Check sheet for the modelled part. Datum: model origin and axes. Units: mm. Round coordinates to 2 decimals unless told otherwise and drop trailing zeros. Answer in a Markdown table with one row per item. Add a question column.
(1) Thickness scan on line 1 along X through (y, z) = (250, -2.9); line 2 along Y through (x, z) = (15, -2.9). Record the ranges inside material, lowest first.
(2) Gauge pin test, flat ends, axial feed: pin 1 (6.5 mm diameter, centred on x = 15, y = 50, fed in from -Z); pin 2 (6.5 mm diameter, centred on x = 15, y = 450, fed in from +Z). Record the tip position at first contact, or that the pin passes through.
(3) Mould release check, pull along Y, two halves, no side actions. Record for faces 1 (the flat face through (217, 254, -3)), 2 (the conical face through (15.63, 47.18, -2.71)): +Y half, -Y half, draft (parallel to the pull), parting line (faces both ways), or undercut.
from build123d import *

# Parameters (mm, degrees)
F0_W           = 440
F0_H           = 500
F1_DEPTH       = 3
F2_D           = 5.5
F2_CSINK_D     = 11.2
F2_CSINK_ANGLE = 90
F3_SIZE        = 5


with BuildPart() as f1:
    # F0 (on Top) → F1 (new body)
    with BuildSketch(Plane.XY):
        with Locations((220, 250)):
            Rectangle(F0_W, F0_H)
    extrude(amount=-F1_DEPTH)

    # F2 (through all)
    with Locations(Plane.XY):
        with Locations((425, 50), (425, 250), (425, 450), (15, 450), (15, 250), (15, 50)):
            CounterSinkHole(F2_D / 2, F2_CSINK_D / 2, counter_sink_angle=F2_CSINK_ANGLE)

    # F3
    f3_edges = [f1.edges().sort_by_distance(p)[0] for p in [
        (0, 0, -1.5),
        (440, 0, -1.5),
        (440, 500, -1.5),
        (0, 500, -1.5),
    ]]
    chamfer(f3_edges, length=F3_SIZE)


solid = f1.part
Answers:
| question | item | result |
|---|---|---|
| 1 | line 1 | x = 0 to 12.25, 17.75 to 422.25, 427.75 to 440 |
| 1 | line 2 | y = 0 to 47.25, 52.75 to 247.25, 252.75 to 447.25, 452.75 to 500 |
| 2 | pin 1 | stops at z = -3 |
| 2 | pin 2 | stops at z = -2.35 |
| 3 | face 1 | draft |
| 3 | face 2 | undercut |
